Could you check a few things on this model? Use its own coordinates, in mm. Face numbers are marked on the shaded views. Round coordinates to 2 decimals unless told otherwise and drop trailing zeros. Loops run counter-clockwise (first coordinate to the right, second up) from the corner with the lowest first, then second, coordinate; pieces in that order, holes last.
from build123d import *

# Parameters (mm, degrees)
F0_W     = 20
F0_H     = 20
F1_DEPTH = 15
F1_TAPER = 3
F2_R     = 2
F4_DEPTH = 3


with BuildPart() as f1:
    # F0 (on Top) → F1 (new body)
    with BuildSketch(Plane.XY):
        with Locations((1.2600612827, 0.3166195687)):
            Rectangle(F0_W, F0_H)
    extrude(amount=F1_DEPTH, taper=F1_TAPER)

    # F2
    f2_edges = [f1.edges().sort_by_distance(p)[0] for p in [
        (-8.34688, 9.923561, 7.5),
        (1.260061, 9.530503, 15),
        (10.473945, 0.31662, 15),
        (1.260061, -8.897264, 15),
        (-7.953822, 0.31662, 15),
        (10.867002, 9.923561, 7.500009),
        (10.867003, -9.290322, 7.5),
        (-8.34688, -9.290322, 7.5),
    ]]
    fillet(f2_edges, radius=F2_R)

    # F3 (on face) → F4 (cut)
    with BuildSketch(Plane.XY.offset(15)):
        Polygon((-4.2536617257, 1.1870977469), (-5.6595876813, 0.7161942194), (-4.2536617257, 0.245290692), (-5.5800070986, -0.1526129199), (-4.3067154475, -0.3913551336), (-5.5800070986, -0.773342629), (-3.3782736864, -0.773342629), (-3.1703652909, -0.1526129199), (-2.9841463782, -0.773342629), (1.2600612827, -0.773342629), (5.5042689435, -0.773342629), (5.6904878563, -0.1526129199), (5.8983962517, -0.773342629), (8.1001296639, -0.773342629), (6.8268380128, -0.3913551336), (8.1001296639, -0.1526129199), (6.773784291, 0.245290692), (8.1797102466, 0.7161942194), (6.773784291, 1.1870977469), (8.1001296639, 1.5850013588), (6.8268380128, 1.8237435725), (8.1001296639, 2.2057310678), (5.8983962517, 2.2057310678), (5.6904878563, 1.5850013588), (5.5042689435, 2.2057310678), (1.2600612827, 2.2057310678), (-2.9841463782, 2.2057310678), (-3.1703652909, 1.5850013588), (-3.3782736864, 2.2057310678), (-5.5800070986, 2.2057310678), (-4.3067154475, 1.8237435725), (-5.5800070986, 1.5850013588), align=None)
    extrude(amount=-F4_DEPTH, mode=Mode.SUBTRACT)


solid = f1.part
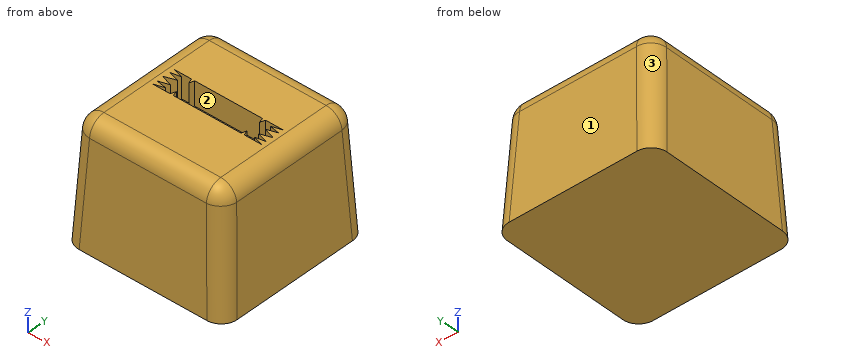
Item 1: If we section it at A-A, the plane x = 4: Please give me the cut outline in (y, z).
Results list:
outline: (-9.68, 0) - (10.32, 0) - (9.63, 13.1) arc R2 ccw to (7.63, 15) - (2.21, 15) - (2.21, 12) - (-0.77, 12) - (-0.77, 15) - (-7, 15) arc R2 ccw to (-9, 13.1) - close
Item 2: Will these pins go through, and if not, where does the flat tip stop? pin 1 (1.5 mm diameter, centred on y = -1.5, z = 8.5, fed in from +X); pin 2 (0.9 mm diameter, centred on x = 1, z = 14, fed in from -Y); pin 3 (1.1 mm diameter, centred on x = 7, z = 13.5, fed in from +Y).
Results list:
pin 1: stops at x = 10.85
pin 2: stops at y = -8.92
pin 3: stops at y = 9.64
Item 3: We'd pull the mould along X, two halves only. Please class the marked faces 1, 2 and 3: released by +X, released by -X, zero draft, split by the parting line, or undercut.
Results list:
face 1: zero draft
face 2: undercut
face 3: released by -X
Item 4: If I drill on line 1 along Z through (x, y) = (-0.25, 1.5); line 2 along Y through (x, z) = (6, 13.75); line 3 along Z through (x, y) = (5.75, 8), over which ranges is the centre line in solid material (lowest first)?
Results list:
line 1: z = 0 to 12
line 2: y = -8.85 to -0.77, 2.21 to 9.49
line 3: z = 0 to 14.97
Item 5: If we section it at B-B, the plane y = -5.25: Please give me the cut outline in (x, z).
Results list:
outline: (-8.74, 0) - (11.26, 0) - (10.57, 13.1) arc R2 ccw to (8.58, 15) - (-6.06, 15) arc R2 ccw to (-8.05, 13.1) - close
